```python
from build123d import *

# Parameters (mm, degrees)
BOSS_EXTRUDE1_DEPTH            = 7.5
BOSS_EXTRUDE2_DEPTH            = 7.5
CUT_EXTRUDE1_DEPTH             = 5
F_3_1_3_1_DIAMETER_HOLE2_D     = 3.1
FILLET1_R                      = 2
FILLET2_R                      = 2
CUT_EXTRUDE2_REACH             = 39.378
CUT_EXTRUDE2_END_RADIUS        = 224.5
SKETCH22_R                     = 2.1
CUT_EXTRUDE2_DIRECTION_2_DEPTH = 0.9
SKETCH23_R                     = 3.5
CUT_EXTRUDE3_DEPTH             = 2.6
SKETCH24_W                     = 2.6
SKETCH24_H                     = 3.5


with BuildPart() as part:
    # Sketch1 → Boss-Extrude1 (new body)
    with BuildSketch(Plane(origin=(0, 0, 0), x_dir=(1, 0, 0), z_dir=(0, 1, 0))):
        with BuildLine():
            ThreePointArc((-207.414551525, 32.851237658), (-210, 0), (-207.414551525, -32.851237658))
            Line((-207.414551525, -32.851237658), (-217.291434931, -34.415582309))
            ThreePointArc((-217.291434931, -34.415582309), (-220, 0), (-217.291434931, 34.415582309))
            Line((-217.291434931, 34.415582309), (-207.414551525, 32.851237658))
        make_face()
        with BuildLine():
            ThreePointArc((-217.291434931, -34.415582309), (-220, 0), (-217.291434931, 34.415582309))
            Line((-217.291434931, 34.415582309), (-220.254499953, 34.884885704))
            ThreePointArc((-220.254499953, 34.884885704), (-223, 0), (-220.254499953, -34.884885704))
            Line((-220.254499953, -34.884885704), (-217.291434931, -34.415582309))
        make_face()
        with BuildLine():
            Line((-204.451486503, 32.381934263), (-207.414551525, 32.851237658))
            ThreePointArc((-207.414551525, 32.851237658), (-210, 0), (-207.414551525, -32.851237658))
            Line((-207.414551525, -32.851237658), (-204.451486503, -32.381934263))
            ThreePointArc((-204.451486503, -32.381934263), (-207, 0), (-204.451486503, 32.381934263))
        make_face()
    extrude(amount=BOSS_EXTRUDE1_DEPTH)

    # Sketch19 → Boss-Extrude2 (add)
    with BuildSketch(Plane(origin=(0, 0, 0), x_dir=(1, 0, 0), z_dir=(0, 1, 0))):
        with BuildLine():
            Line((-224.019328267, 14.683002512), (-222.522539882, 14.584897818))
            ThreePointArc((-222.522539882, 14.584897818), (-223, 0), (-222.522539882, -14.584897818))
            Line((-222.522539882, -14.584897818), (-224.019328267, -14.683002512))
            ThreePointArc((-224.019328267, -14.683002512), (-224.5, 0), (-224.019328267, 14.683002512))
        make_face()
    extrude(amount=BOSS_EXTRUDE2_DEPTH)

    # Sketch15 → Cut-Extrude1 (cut)
    with BuildSketch(Plane(origin=(0, 7.5, 0), x_dir=(1, 0, 0), z_dir=(0, 1, 0))):
        with BuildLine():
            Line((-219.772609758, 10), (-209.761769634, 10))
            ThreePointArc((-209.761769634, 10), (-208.900850883, 21.457737542), (-207.414551525, 32.851237658))
            Line((-207.414551525, 32.851237658), (-217.291434931, 34.415582309))
            ThreePointArc((-217.291434931, 34.415582309), (-218.872736893, 22.242415451), (-219.772609758, 10))
        make_face()
        with BuildLine():
            ThreePointArc((-207.414551525, -32.851237658), (-208.900850883, -21.457737542), (-209.761769634, -10))
            Line((-209.761769634, -10), (-219.772609758, -10))
            ThreePointArc((-219.772609758, -10), (-218.872736893, -22.242415451), (-217.291434931, -34.415582309))
            Line((-217.291434931, -34.415582309), (-207.414551525, -32.851237658))
        make_face()
    extrude(amount=-CUT_EXTRUDE1_DEPTH, mode=Mode.SUBTRACT)

    # Ø3.1 (3.1) Diameter Hole2 (through all)
    with Locations(Plane(origin=(0, 0, 0), x_dir=(-1, 0, 0), z_dir=(0, -1, 0))):
        with Locations((213.160645195, -28.063131327), (214.18186009, -18.738484691), (214.18186009, 18.738484691), (213.160645195, 28.063131327)):
            Hole(F_3_1_3_1_DIAMETER_HOLE2_D / 2)

    # Fillet1
    fillet1_edges = [part.edges().sort_by_distance(p)[0] for p in [
        (-220.254499953, 3.75, 34.884885704),
        (-220.254499953, 3.75, -34.884885704),
        (-204.451486503, 3.75, -32.381934263),
        (-204.451486503, 3.75, 32.381934263),
    ]]
    fillet(fillet1_edges, radius=FILLET1_R)

    # Fillet2
    # the kernel refuses this fillet: 2 mm, written as the material it adds along each edge
    with BuildSketch(Plane(origin=(-222.522539882, 0, -14.584897818), x_dir=(0.06970140258603677, 0, -0.9975678996827931), z_dir=(0, 1, 0))) as fillet2_piece_1:
        with BuildLine():
            CenterArc((1.930030715, 1.99998144), FILLET2_R, 194.477374901, 75.275788142)
            Line((-0.006462156, 1.49998608), (-0.045192014, 1.489986173))
            ThreePointArc((-0.045192014, 1.489986173), (-0.043230707, 0.749820716), (-0.039999629, -0.000172324))
            Line((-0.039999629, -0.000172324), (0.000172324, -0.039999629))
            ThreePointArc((0.000172324, -0.039999629), (0.960707253, -0.037930577), (1.921242182, -0.039999629))
            Line((1.921242182, -0.039999629), (1.921414506, 0))
        make_face()
    extrude(amount=7.5)
    with BuildSketch(Plane(origin=(-222.522539882, 0, 14.584897818), x_dir=(-0.9978589232386029, 0, 0.06540312923015226), z_dir=(0, 1, 0))) as fillet2_piece_2:
        with BuildLine():
            CenterArc((1.991648107, 1.938628933), FILLET2_R, 180.493673912, 75.275788142)
            Line((-0.008277654, 1.921396676), (-0.048276169, 1.92105203))
            ThreePointArc((-0.048276169, 1.92105203), (-0.042069052, 0.960534929), (-0.04, 0))
            Line((-0.04, 0), (0, -0.04))
            ThreePointArc((0, -0.04), (0.75, -0.04), (1.490167038, -0.038772579))
            Line((1.490167038, -0.038772579), (1.5, 0))
        make_face()
    extrude(amount=7.5)

    # Cut-Extrude2: up to this cylinder (the profile starts inside it)
    cut_extrude2_end = Plane(origin=(0, 7.5, 0), z_dir=(0, -1, 0)) * Cylinder(CUT_EXTRUDE2_END_RADIUS, 528.756, mode=Mode.PRIVATE)
    # Sketch22 → Cut-Extrude2 (cut, up to the surface)
    with BuildSketch(Plane(origin=(-212.5, 0, 0), x_dir=(0, 0, -1), z_dir=(1, 0, 0)), mode=Mode.PRIVATE) as cut_extrude2_sk1:
        with Locations((0, 7.5)):
            Circle(SKETCH22_R)
    cut_extrude2_tool1 = extrude(cut_extrude2_sk1.sketch, amount=-CUT_EXTRUDE2_REACH, mode=Mode.PRIVATE) & cut_extrude2_end
    add(cut_extrude2_tool1.solids().sort_by_distance((-212.5, 7.5, 0))[0], mode=Mode.SUBTRACT)

    # Sketch22 → Cut-Extrude2 direction 2 (cut)
    with BuildSketch(Plane(origin=(-212.5, 0, 0), x_dir=(0, 0, -1), z_dir=(1, 0, 0))):
        with Locations((0, 7.5)):
            Circle(SKETCH22_R)
    extrude(amount=CUT_EXTRUDE2_DIRECTION_2_DEPTH, mode=Mode.SUBTRACT)

    # Sketch23 → Cut-Extrude3 (cut)
    with BuildSketch(Plane.ZY.offset(211.6)):
        with Locations((0, 7.439199918)):
            Circle(SKETCH23_R)
    extrude(amount=CUT_EXTRUDE3_DEPTH, mode=Mode.SUBTRACT)

    # Sketch24 → Cut-Revolve1 (revolve, cut)
    with BuildSketch(Plane(origin=(0, 7.5, 0), x_dir=(1, 0, 0), z_dir=(0, 1, 0))):
        with Locations((-223.2, 1.75)):
            Rectangle(SKETCH24_W, SKETCH24_H)
    revolve(axis=Axis((-224.5, 7.5, 0), (1, 0, 0)), mode=Mode.SUBTRACT)


solid = part.part
```
The listing builds one solid part. Answer for the finished solid, in the listing's coordinates (mm). A direction names the side the tool comes from. Coordinates: 2 decimals unless noted, no trailing zeros. Loops run counter-clockwise (first coordinate to the right, second up) from the corner with the lowest first, then second, coordinate; pieces in that order, holes last. Notation, with made-up numbers: (76.25, -12) -> (89.25, -12) arc R30 cw to (89.25, 17) -> close; hole circle Ø11 at (-14.5, -27.75). An arc over 180 degrees is marked (long way). Return JSON: item names as keys, results as strings. Group by question number.
(1) Determine the mould class of faces 1 (the cylindrical face through (-218.855, 5.035, -22.413)), 2 (the cylindrical face through (-223, 4, 0)), 3 (the cylindrical face through (-221.64, 3.7, 24.6)), 4 (the cylindrical face through (-208.917, 5.035, -21.298)) for opening direction Z: released by +Z, released by -Z, zero draft, split by the parting line, or undercut.
(2) Given pin 1 Ø1.5 at (x, y) = (-221, 1.5) entering from +Z; pin 2 Ø1.5 at (x, y) = (-217, 5) entering from -Z; pin 3 Ø1 at (y, z) = (2, -15.5) entering from -X, each flat-ended and moving along its own axis, determine where each tip first touches the part or whether it passes through.
(3) A cutting plane is placed at A-A on z = 0. Write down the section's boundary in (x, y).
(4) Which of the six approach directions +Z, -Z, +X, -X, +Y, -Y give full straight-line access (tool end or side, diameter ignored) to faces 5 (the flat face through (-221.9, 5, 0)), 6 (the flat face through (-214.2, 5, 0)), 7 (the cylindrical face through (-207, 4, 0))?
(5) A cutting plane is placed at B-B on z = -19.5. Write down the section's boundary in (x, y).
(6) Find the intervals of material crossed by probe 1 along Z at (x, y) = (-212.5, 1); probe 2 along Y at (x, z) = (-216.5, 28); probe 3 along Z at (x, y) = (-216, 3.25), in increasing order. Write a range as from..to.
(7) A cutting plane is placed at C-C on y = 1.5. Write down the section's boundary in (x, z), and give its area (3 significant figures).
The answers:
{
 "1": {"face 1": "undercut", "face 2": "undercut", "face 3": "released by +Z", "face 4": "released by -Z"},
 "2": {"pin 1": "stops at z = 33.7", "pin 2": "stops at z = -34.49", "pin 3": "stops at x = -223.25"},
 "3": {"outline": "(-224.5, 0) -> (-207, 0) -> (-207, 7.5) -> (-211.6, 7.5) -> (-211.6, 3.94) -> (-214.2, 3.94) -> (-214.2, 5.4) -> (-221.9, 5.4) -> (-221.9, 4) -> (-224.5, 4) -> close"},
 "4": {"face 5": "-X, +Y", "face 6": "+Y", "face 7": "+X, +Y, -Y"},
 "5": {"outline": "(-222.15, 0) -> (-215.53, 0) -> (-215.53, 2.5) -> (-219.13, 2.5) -> (-219.13, 7.5) -> (-222.15, 7.5) -> close; (-212.83, 0) -> (-206.08, 0) -> (-206.08, 7.5) -> (-209.09, 7.5) -> (-209.09, 2.5) -> (-212.83, 2.5) -> close"},
 "6": {"probe 1": "z = -33.66..-29.47, -26.66..26.66, 29.47..33.66", "probe 2": "y = 0..2.5", "probe 3": "z = -10..10"},
 "7": {"outline": "(-224.02, -14.68) arc R2 cw to (-222.39, -16.5) arc R223 ccw to (-220.56, -32.89) arc R2 ccw to (-218.27, -34.57) -> (-206.42, -32.69) arc R2 ccw to (-204.75, -30.42) arc R207 cw to (-204.75, 30.42) arc R2 ccw to (-206.42, 32.69) -> (-218.27, 34.57) arc R2 ccw to (-220.56, 32.89) arc R223 ccw to (-222.39, 16.5) arc R2 cw to (-224.02, 14.68) arc R224.5 ccw to start; hole circle Ø3.1 at (-214.18, -18.74); hole circle Ø3.1 at (-214.18, 18.74); hole circle Ø3.1 at (-213.16, -28.06); hole circle Ø3.1 at (-213.16, 28.06)", "area": "1,090 mm^2"}
}
